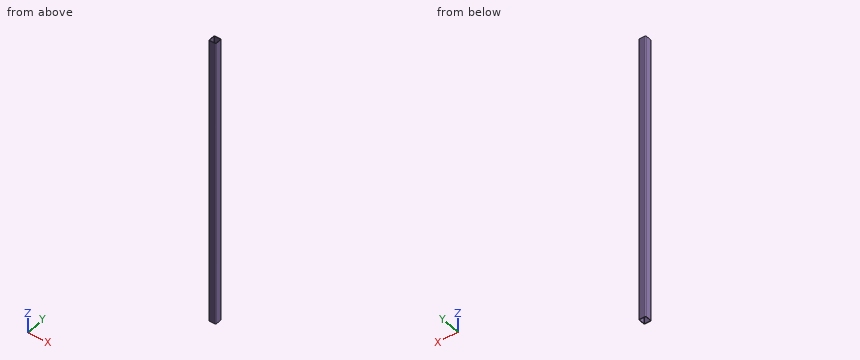
Autodesk Inventor part; units mm, degrees
ref_plane "Plano inicial" through (0, 0, 25.4) normal (0, 0, 1) x (1, 0, 0)
ref_plane "Plano final" through (0, 0, 2064.6) normal (0, 0, 1) x (1, 0, 0)
ref_plane "Plano de trabajo4" through (-19.05, 1700, 25.4) normal (0, 0, -1) x (-1, 0, 0)
ref_plane "Plano inicial" through (0, 0, 25.4) normal (0, 0, 1) x (1, 0, 0)
ref_plane "Plano final" through (0, 0, 2064.6) normal (0, 0, 1) x (1, 0, 0)
sketch "Boceto" plane through (0, 0, 0) normal (0, 0, 1) x (1, 0, 0)
  line L0 (-25.4, -19.05) -> (-25.4, 19.05)
  line L1 (-19.05, 25.4) -> (19.05, 25.4)
  line L2 (25.4, 19.05) -> (25.4, -19.05)
  line L3 (19.05, -25.4) -> (-19.05, -25.4)
  arc A0 (-25.4, -19.05) -> (-19.05, -25.4) centre (-19.05, -19.05) ccw
  arc A1 (-19.05, 25.4) -> (-25.4, 19.05) centre (-19.05, 19.05) ccw
  arc A2 (25.4, 19.05) -> (19.05, 25.4) centre (19.05, 19.05) ccw
  arc A3 (19.05, -25.4) -> (25.4, -19.05) centre (19.05, -19.05) ccw
  arc A4 (-19.05, 22.225) -> (-22.225, 19.05) centre (-19.05, 19.05) ccw
  line L4 (-19.05, 22.225) -> (19.05, 22.225)
  arc A5 (22.225, 19.05) -> (19.05, 22.225) centre (19.05, 19.05) ccw
  line L5 (22.225, 19.05) -> (22.225, -19.05)
  arc A6 (19.05, -22.225) -> (22.225, -19.05) centre (19.05, -19.05) ccw
  line L6 (19.05, -22.225) -> (-19.05, -22.225)
  arc A7 (-22.225, -19.05) -> (-19.05, -22.225) centre (-19.05, -19.05) ccw
  line L7 (-22.225, -19.05) -> (-22.225, 19.05)
  line L8 (0, 37.4012) -> (0, -37.4012) construction
  line L9 (-37.4012, 0) -> (37.4012, 0) construction
  dimension "d10" = 50.8
  dimension "d11" = 50.8
  dimension "d12" = 3.175
  dimension "d15" = 25.4
  dimension "d16" = 25.4
  dimension "d17" = 6.35
extrude "Cuerpo" add sketch "Boceto" along normal up to surface (2039.2 mm away) from surface at 25.4
sketch "Sketch3" plane through (0, 0, 0) normal (0, 0, 1) x (1, 0, 0)
  line L0 (0, 0) -> (10, 0)
ref_plane "Work Plane3" through (0, 0, 0) normal (0, -1, 0) x (1, 0, 0)
ref_plane "Plano de trabajo4" through (-19.05, 1700, 25.4) normal (0, 0, -1) x (-1, 0, 0)
split "Dividir1" plane through (-19.05, 1700, 25.4) removes the side toward (0, 0, -1)
ref_plane "Plano de trabajo5" through (19.05, 1700, 2064.6) normal (0, 0, 1) x (1, 0, 0)
split "Dividir2" plane through (19.05, 1700, 2064.6) removes the side toward (0, 0, 1)
sketch "Sketch4" plane through (0, 0, 0) normal (0, -1, 0) x (1, 0, 0)
  line L0 (-2, 25.4) -> (12, 25.4)
  line L1 (-2, 2064.6) -> (12, 2064.6)
  dimension "d19" = 2039.2
equation "\"d10\" = G_H"
equation "\"d11\" = G_W"
equation "\"d12\" = G_T"
equation "\"d15\" = 0.5 * d10"
equation "\"d16\" = 0.5 * d11"
equation "\"d17\" = G_IR"
equation "\"d3\" = G_L"
equation "\"G_W\" = 50.8"
equation "\"G_H\" = 50.8"
equation "\"G_T\" = 3.175"
equation "\"G_IR\" = 6.35"
equation "\"G_L\" = d19"
equation "\"G_OFFSET_START\" = -25.4"
equation "\"G_OFFSET_END\" = -25.4"
equation "\"d13\" = -G_OFFSET_START"
equation "\"d14\" = G_OFFSET_END + B_L"
equation "\"B_L\" = 2090"
properties part number "AISC - 2 x 2 x 1/8 - 80,283" material "Acero, suave"
Source: CAD feature listing. Evaluate the final solid. Frame: model axes, mm. Give positions to 0.01 mm unless a question says otherwise; leave off trailing zeros. Loops run counter-clockwise (first coordinate to the right, second up) from the corner with the lowest first, then second, coordinate; pieces in that order, holes last. Notation, with made-up numbers: M -13,-9 L -5,-9 A24 ccw -5,10 Z; hole C -5.75,-14 d6. An arc over 180 degrees is marked long. Put each result on its own line as item: value.
Q1. Section A-A (y = -2). Return the cut outline in (x, z) (3 decimals), and give its area (3 significant figures).
Response values:
outline: M -25.4,25.4 L -22.225,25.4 L -22.225,2064.6 L -25.4,2064.6 Z; M 22.225,25.4 L 25.4,25.4 L 25.4,2064.6 L 22.225,2064.6 Z
area: 12,900 mm²
Q2. Section C-C (z = 890). Return the cut outline in (x, y) (3 decimals), and give its area (3 significant figures).
Response values:
outline: M -25.4,-19.05 A6.35 ccw -19.05,-25.4 L 19.05,-25.4 A6.35 ccw 25.4,-19.05 L 25.4,19.05 A6.35 ccw 19.05,25.4 L -19.05,25.4 A6.35 ccw -25.4,19.05 Z; hole M -22.225,-19.05 A3.175 ccw -19.05,-22.225 L 19.05,-22.225 A3.175 ccw 22.225,-19.05 L 22.225,19.05 A3.175 ccw 19.05,22.225 L -19.05,22.225 A3.175 ccw -22.225,19.05 Z
area: 579 mm²
Q3. Pin query (flat end, axial travel): P1, Ø10, axis at x = -14, y = 11.5, coming from the +Z side. Return the tip coordinate at first contact, or that it passes through.
Response values:
P1: passes through
Q4. Line query: probe 1 along X at (y, z) = (-20.5, 1411); probe 2 along X at (y, z) = (-6, 1921) (3 decimals). Output: solid intervals per line, ascending. Write a range as [from, to].
Response values:
probe 1: x = [-25.23, -21.87], [21.87, 25.23]
probe 2: x = [-25.4, -22.225], [22.225, 25.4]
